```python
from build123d import *

# Parameters (mm, degrees)
F1_DEPTH = 5
F0_W     = 7.9375
F0_H     = 2.5
F2_DEPTH = 1
F3_DEPTH = 3.175


with BuildPart() as f1:
    # F0 (on Top) → F1 (new body)
    with BuildSketch(Plane.XY):
        Polygon((7.5, 6), (7.5, -6), (7.5, -7.5875), (9.0875, -7.5875), (9.0875, 6), align=None)
        Polygon((7.5, -7.5875), (7.5, -6), (4.5, -6), (-7.5, -6), (-7.5, -7.5875), align=None)
        Polygon((-7.5, -7.5875), (-7.5, -6), (-7.5, 4.4125), (-7.5, 6), (-7.5875, 6), (-9.0875, 6), (-9.0875, -7.5875), align=None)
    extrude(amount=F1_DEPTH)

    # F0 (on Top) → F2 (join)
    with BuildSketch(Plane.XY):
        Polygon((7.5, -7.5875), (7.5, -6), (4.5, -6), (-7.5, -6), (-7.5, -7.5875), align=None)
        Polygon((4.5, -6), (7.5, -6), (7.5, 6), (3.96875, 6), (3.96875, 3.5), (-3.96875, 3.5), (-3.96875, 6), (-5.46875, 6), (-6, 6), (-7.5, 6), (-7.5, 4.4125), (-7.5, -6), align=None)
        Polygon((7.5, 6), (7.5, -6), (7.5, -7.5875), (9.0875, -7.5875), (9.0875, 6), align=None)
        Polygon((-7.5, -7.5875), (-7.5, -6), (-7.5, 4.4125), (-7.5, 6), (-7.5875, 6), (-9.0875, 6), (-9.0875, -7.5875), align=None)
        with Locations((0, 4.75)):
            Rectangle(F0_W, F0_H)
    extrude(amount=F2_DEPTH)

    # F0 (on Top) → F3 (join)
    with BuildSketch(Plane.XY):
        with Locations((0, 4.75)):
            Rectangle(F0_W, F0_H)
    extrude(amount=-F3_DEPTH)


solid = f1.part
```
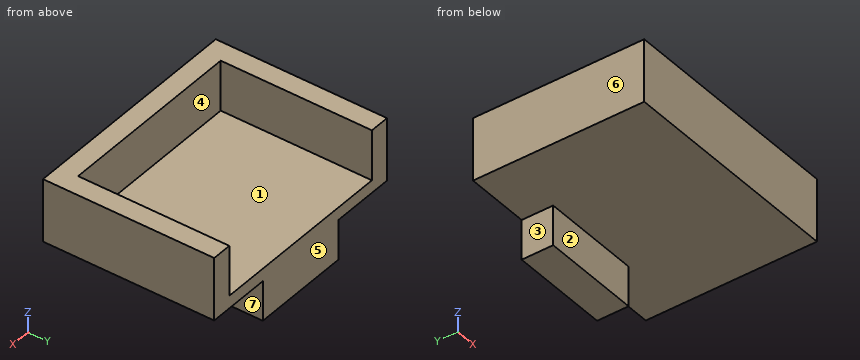
Read the model definition and answer for the solid it produces. Units are mm, in the model's axes. Face numbers are marked on the shaded views. A direction names the side the tool comes from. Coordinates: 2 decimals unless noted, no trailing zeros. Order: outer loops, then holes, each group sorted by start corner. A loop starts at its lowest first (then second) coordinate and runs counter-clockwise, first axis right, second up. Notation, with made-up numbers: (-5, 38.5) - (21, 38.5) arc R11 cw to (21, 44.5) - close; hole circle Ø2 at (40, 26.25). An arc over 180 degrees is marked (long way). Answer as a JSON object with one key per item and string values. Group by question number.
Item 1: Flat-ended cylindrical pins translate along their axes: P1, Ø4.5, axis at x = 1, z = 2.5, coming from the +Y side; P2, Ø6, axis at x = 2.5, y = -1.5, coming from the +Z side; P3, Ø1.2, axis at y = 4.5, z = -2, coming from the +X side; P4, Ø1, axis at x = 5.5, y = -2, coming from the -Z side. Find the tip coordinate at first contact, or state that the pin passes through.
Item 2: Section C-C (z = 3) is taken. Give the vertices of the cut face in (x, y), plus the area to 3 significant figures.
Item 3: The mould has two halves that part along X. Classify the marked faces 4, 5, 6 and 7: +X half, -X half, draft (parallel to the pull), parting line (faces both ways), or undercut.
Item 4: Consider probe 1 along X at (y, z) = (1, 2.5); probe 2 along Z at (x, y) = (-6.75, 1.25); probe 3 along X at (y, z) = (5, -0.75). Determine where each line is inside the solid, lowest interval first. Write a range as from..to.
Item 5: Section A-A (x = 5.25) is taken. Give the vertices of the cut face in (y, z).
Item 6: Section B-B (y = -5) is taken. Give the vertices of the cut face in (x, z), plus the area to 3 significant figures.
Item 7: Section D-D (z = -2.5) is taken. Give the vertices of the cut face in (x, y), plus the area to 3 significant figures.
Item 8: A tool of negligible diameter and unlimited length cuts with its end or side. For the marked faces 1, 2 and 3, from which of +Z, -Z, +X, -X, +Y, -Y can it reach the whole face along a straight path? Write none if from no direction.
Results are:
{
 "1": {"P1": "stops at y = 6", "P2": "stops at z = 1", "P3": "stops at x = 3.97", "P4": "stops at z = 0"},
 "2": {"outline": "(-9.09, -7.59) - (9.09, -7.59) - (9.09, 6) - (7.5, 6) - (7.5, -6) - (-7.5, -6) - (-7.5, 6) - (-9.09, 6) - close", "area": "67.0 mm^2"},
 "3": {"face 4": "undercut", "face 5": "draft", "face 6": "-X half", "face 7": "+X half"},
 "4": {"probe 1": "x = -9.09..-7.5, 7.5..9.09", "probe 2": "z = 0..1", "probe 3": "x = -3.97..3.97"},
 "5": {"outline": "(-7.59, 0) - (6, 0) - (6, 1) - (-6, 1) - (-6, 5) - (-7.59, 5) - close"},
 "6": {"outline": "(-9.09, 0) - (9.09, 0) - (9.09, 5) - (7.5, 5) - (7.5, 1) - (-7.5, 1) - (-7.5, 5) - (-9.09, 5) - close", "area": "30.9 mm^2"},
 "7": {"outline": "(-3.97, 3.5) - (3.97, 3.5) - (3.97, 6) - (-3.97, 6) - close", "area": "19.8 mm^2"},
 "8": {"face 1": "+Z, +Y", "face 2": "-Z, +X, -X, -Y", "face 3": "-Z, -X, +Y, -Y"}
}
